Print and shaded views of the part. All mm, measured from the part's lowest x, y and z. Give positions to 0.01 mm unless a question says otherwise; leave off trailing zeros. Order: outer loops, then holes, each group sorted by start corner. A loop starts at its lowest first (then second) coordinate and runs counter-clockwise, first axis right, second up. Notation, with made-up numbers: (35.25, 41) - (88.25, 41) arc R25 cw to (88.25, 54) - close; hole circle Ø11 at (-34, 23.5). An arc over 180 degrees is marked (long way). Answer in a Markdown table with one row per item.
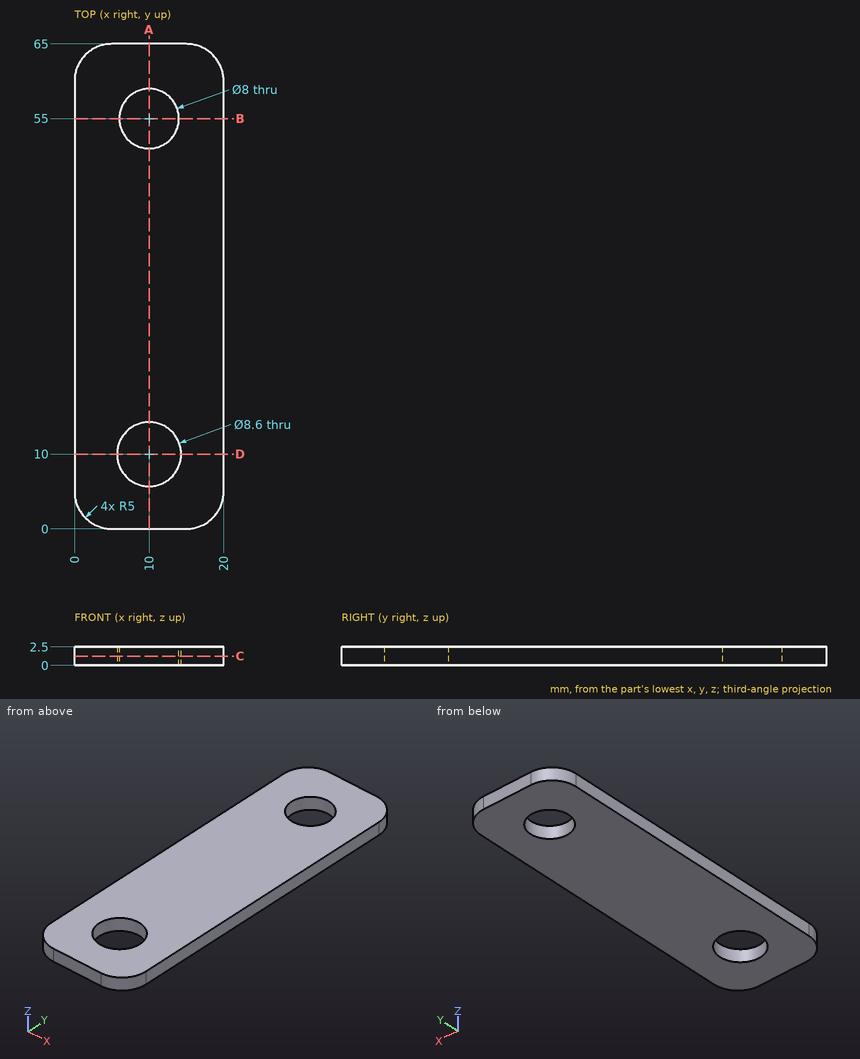
1. Drop a flat-ended pin along its axis: P1, Ø7, axis at x = 10, y = 10, coming from the +Z side. Give the stop position or say it passes through.
Check result:
| item | result |
|---|---|
| P1 | passes through |
2. Cut at A-A on x = 10. Write the cut outline in (y, z).
Check result:
| item | result |
|---|---|
| outline | (0, 0) - (5.7, 0) - (5.7, 2.5) - (0, 2.5) - close; (14.3, 0) - (51, 0) - (51, 2.5) - (14.3, 2.5) - close; (59, 0) - (65, 0) - (65, 2.5) - (59, 2.5) - close |
3. Cut at C-C on z = 1.25. Write the cut outline in (x, y).
Check result:
| item | result |
|---|---|
| outline | (0, 5) arc R5 ccw to (5, 0) - (15, 0) arc R5 ccw to (20, 5) - (20, 60) arc R5 ccw to (15, 65) - (5, 65) arc R5 ccw to (0, 60) - close; hole circle Ø8.6 at (10, 10); hole circle Ø8 at (10, 55) |
4. Probe line 1 (Y direction, x = 10, z = 0.9); line 2 (Y direction, x = 12.5, z = 0.45); line 3 (Y direction, x = 3, z = 1.75). List the from-to ranges inside material, lowest first.
Check result:
| item | result |
|---|---|
| line 1 | y = 0 to 5.7, 14.3 to 51, 59 to 65 |
| line 2 | y = 0 to 6.5, 13.5 to 51.88, 58.12 to 65 |
| line 3 | y = 0.42 to 64.58 |
5. Cut at B-B on y = 55. Write the cut outline in (x, z).
Check result:
| item | result |
|---|---|
| outline | (0, 0) - (6, 0) - (6, 2.5) - (0, 2.5) - close; (14, 0) - (20, 0) - (20, 2.5) - (14, 2.5) - close |
6. Cut at D-D on y = 10. Write the cut outline in (x, z), and give its area (3 significant figures).
Check result:
| item | result |
|---|---|
| outline | (0, 0) - (5.7, 0) - (5.7, 2.5) - (0, 2.5) - close; (14.3, 0) - (20, 0) - (20, 2.5) - (14.3, 2.5) - close |
| area | 28.5 mm² |
